Source: three-view drawing plus pictorial views. Frame: mm from the lowest corner of the part. A direction names the side the tool comes from. Give positions to 0.01 mm unless a question says otherwise; leave off trailing zeros. Write each loop counter-clockwise with the first axis right and the second up, starting at its lowest first coordinate (ties: lowest second). Pieces come first, ordered by that corner, then holes.
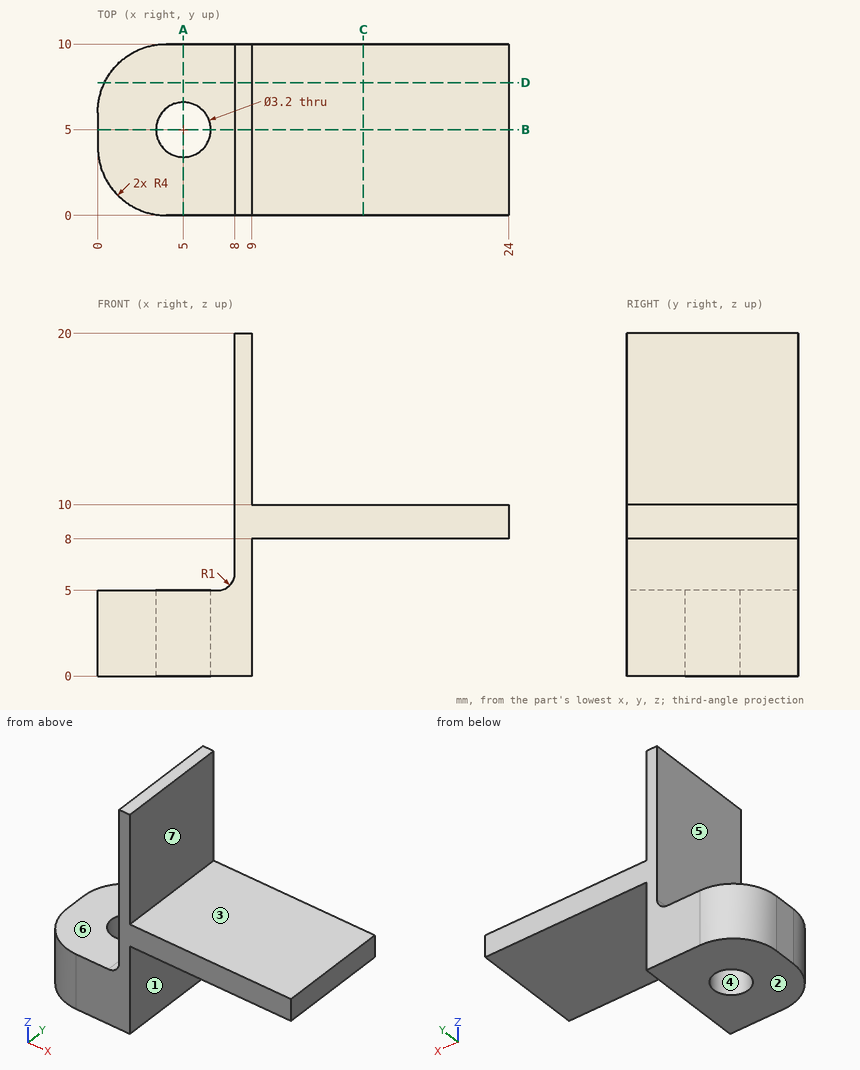
Q1. Ray query, line 1 along X through (y, z) = (5, 1.5); line 2 along Y through (x, z) = (5, 3.3); line 3 along X through (y, z) = (4.5, 7.5). Return the intervals inside material, ascending.
Filled sheet:
line 1: x = 0 to 3.4, 6.6 to 9
line 2: y = 0 to 3.4, 6.6 to 10
line 3: x = 8 to 9
Q2. Pin query (flat end, axial travel): P1, Ø2.5, axis at x = 5, y = 5, coming from the -Z side; P2, Ø3, axis at x = 7.5, y = 7.5, coming from the -Z side; P3, Ø3, axis at y = 3.5, z = 14, coming from the +X side; P4, Ø3, axis at x = 5.5, y = 4, coming from the +Z side. Return the tip coordinate at first contact, or that it passes through.
Filled sheet:
P1: passes through
P2: stops at z = 0
P3: stops at x = 9
P4: stops at z = 5
Q3. Section D-D on y = 7.75. Output: boundary loops of the cut face in (x, z).
Filled sheet:
outline: (0.4, 0) - (9, 0) - (9, 8) - (24, 8) - (24, 10) - (9, 10) - (9, 20) - (8, 20) - (8, 6) arc R1 cw to (7, 5) - (0.4, 5) - close
Q4. Section B-B on y = 5. Output: boundary loops of the cut face in (x, z).
Filled sheet:
outline: (0, 0) - (3.4, 0) - (3.4, 5) - (0, 5) - close; (6.6, 0) - (9, 0) - (9, 8) - (24, 8) - (24, 10) - (9, 10) - (9, 20) - (8, 20) - (8, 6) arc R1 cw to (7, 5) - (6.6, 5) - close
Q5. Access query for the marked faces 1, 2 and 3. Directions: +Z, -Z, +X, -X, +Y, -Y. A direction counts if a zero-diameter tool reaches every point of the face in a straight line with its end or side. Return the directions, or none.
Filled sheet:
face 1: -Z, +X, +Y, -Y
face 2: -Z, +X, -X, +Y, -Y
face 3: +Z, +X, +Y, -Y
Q6. Section C-C on x = 15.5. Output: boundary loops of the cut face in (y, z).
Filled sheet:
outline: (0, 8) - (10, 8) - (10, 10) - (0, 10) - close
Q7. Section A-A on x = 5. Output: boundary loops of the cut face in (y, z).
Filled sheet:
outline: (0, 0) - (3.4, 0) - (3.4, 5) - (0, 5) - close; (6.6, 0) - (10, 0) - (10, 5) - (6.6, 5) - close
Q8. Pull-direction query (X, two-part tool) for the marked faces 4, 5, 6 and 7; classes: released by +X, released by -X, zero draft, split by the parting line, or undercut.
Filled sheet:
face 4: undercut
face 5: released by -X
face 6: zero draft
face 7: released by +X
